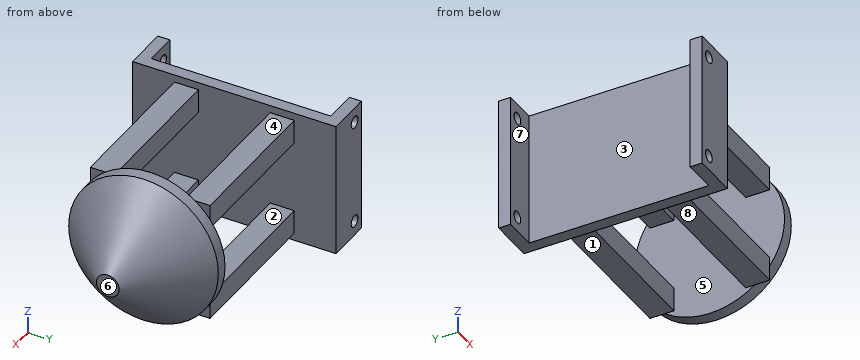
Autodesk Fusion 360 part; units mm, degrees
sketch "Sketch1" plane through (0, 0, 0) normal (0, 1, 0) x (1, 0, 0)
  line L0 (7.5, -22.5) -> (-7.5, -22.5)
  line L1 (-7.5, -22.5) -> (-7.5, 22.5)
  line L2 (-7.5, 22.5) -> (7.5, 22.5)
  line L3 (7.5, 22.5) -> (7.5, -22.5)
  line L4 (7.5, -22.5) -> (-7.5, 22.5) construction
  line L5 (-7.5, -22.5) -> (7.5, 22.5) construction
  dimension "d1" = 45
  dimension "d2" = 15
extrude "Extrude1" add sketch "Sketch1" along normal blind 4
sketch "Sketch2" plane through (0, 4, 0) normal (0, 1, 0) x (-1, 0, 0)
  line L0 (-7.5, -22.5) -> (7.5, -22.5)
  line L1 (7.5, -22.5) -> (7.5, 22.5)
  line L2 (7.5, 22.5) -> (-7.5, 22.5)
  line L3 (-7.5, 22.5) -> (-7.5, -22.5)
  line L4 (-7.5, 22.5) -> (-3.5, 22.5)
  line L5 (-3.5, 22.5) -> (-3.5, -22.5)
  line L6 (-3.5, -22.5) -> (-7.5, -22.5)
  line L7 (-7.5, -22.5) -> (-7.5, 22.5)
  dimension "d9" = 4
extrude "Extrude2" add sketch "Sketch2" along normal blind 64 contours L0 L2 L3 L4 L5 L6 L7
sketch "Sketch3" plane through (3.5, 0, 0) normal (-1, 0, 0) x (0, -1, 0)
  line L0 (-4, -22.5) -> (-4, 22.5)
  line L1 (-4, 22.5) -> (-68, 22.5)
  line L2 (-68, 22.5) -> (-68, -22.5)
  line L3 (-68, -22.5) -> (-4, -22.5)
  line L4 (-68, 22.5) -> (-64, 22.5)
  line L5 (-64, 22.5) -> (-64, -22.5)
  line L6 (-64, -22.5) -> (-68, -22.5)
  line L7 (-68, -22.5) -> (-68, 22.5)
  dimension "d12" = 4
extrude "Extrude3" add sketch "Sketch3" along normal blind 11 contours L1 L2 L3 L4 L5 L6 L7
sketch "Sketch4" plane through (3.5, 0, 0) normal (-1, 0, 0) x (0, -1, 0)
  line L0 (-64, 22.5) -> (-64, -22.5)
  line L1 (-64, -22.5) -> (-4, -22.5)
  line L2 (-4, -22.5) -> (-4, 22.5)
  line L3 (-4, 22.5) -> (-64, 22.5)
  line L4 (-60, 22.5) -> (-56, 22.5)
  line L5 (-56, 22.5) -> (-56, -22.5)
  line L6 (-56, -22.5) -> (-60, -22.5)
  line L7 (-60, -22.5) -> (-60, 22.5)
  line L8 (-34, -22.5) -> (-34, 22.5) construction
  line L9 (-8, 22.5) -> (-12, 22.5)
  line L10 (-8, -22.5) -> (-8, 22.5)
  line L11 (-12, 22.5) -> (-12, -22.5)
  line L12 (-12, -22.5) -> (-8, -22.5)
  dimension "d15" = 4
  dimension "d16" = 4
sketch "Sketch5" plane through (0, 68, 0) normal (0, 1, 0) x (-1, 0, 0)
  line L0 (-7.5, -22.5) -> (7.5, -22.5)
  line L1 (7.5, -22.5) -> (7.5, 22.5)
  line L2 (7.5, 22.5) -> (-7.5, 22.5)
  line L3 (-7.5, 22.5) -> (-7.5, -22.5)
  circle A0 centre (3.5, 17.4201) radius 2
  circle A1 centre (3.5, -17.5799) radius 2
  line L4 (3.5, -17.5799) -> (3.5, 17.4201) construction
  point P0 (3.5, -0.0799)
  dimension "d19" = 4
  dimension "d20" = 4
  dimension "d21" = 35
  dimension "d22" = 4
extrude "Extrude5" cut sketch "Sketch5" against normal through all contours A0 | A1
ref_plane "WorkPlane1" through (0, 34, 0) normal (0, 1, 0) x (0, 0, 1)
sketch "Sketch7" plane through (7.5, 0, 0) normal (1, 0, 0) x (0, 1, 0)
  line L0 (0, 22.5) -> (0, -22.5)
  line L1 (0, -22.5) -> (68, -22.5)
  line L2 (68, -22.5) -> (68, 22.5)
  line L3 (68, 22.5) -> (0, 22.5)
  line L4 (54, 20) -> (14, 20) construction
  line L5 (14, 20) -> (14, -20) construction
  line L6 (14, -20) -> (54, -20) construction
  line L7 (54, -20) -> (54, 20) construction
  line L8 (54, 20) -> (14, -20) construction
  line L9 (14, 20) -> (54, -20) construction
  line L10 (34, 22.5) -> (34, -22.5) construction
  line L11 (0, 0) -> (68, 0) construction
  line L12 (14, 20) -> (22, 20)
  line L13 (22, 20) -> (22, 12)
  line L14 (22, 12) -> (14, 12)
  line L15 (14, 12) -> (14, 20)
  line L16 (46, 12) -> (54, 12)
  line L17 (54, 12) -> (54, 20)
  line L18 (54, 20) -> (46, 20)
  line L19 (46, 20) -> (46, 12)
  line L20 (22, -12) -> (14, -12)
  line L21 (22, -20) -> (22, -12)
  line L22 (14, -20) -> (22, -20)
  line L23 (14, -12) -> (14, -20)
  line L24 (46, -20) -> (46, -12)
  line L25 (54, -20) -> (46, -20)
  line L26 (54, -12) -> (54, -20)
  line L27 (46, -12) -> (54, -12)
  point P0 (34, 0)
  dimension "d32" = 40
  dimension "d33" = 40
  dimension "d34" = 8
extrude "Extrude6" add sketch "Sketch7" along normal blind 50 contours L12 L13 L14 L15 | L16 L17 L18 L19 | L20 L21 L22 L23 | L24 L25 L26 L27
sketch "Sketch8" plane through (0, 34, 0) normal (0, 1, 0) x (1, 0, 0)
  line L0 (57.5, -20) -> (57.5, -12)
  line L1 (0, 0) -> (67.5, 0) construction
  line L2 (57.5, -25) -> (61.5, -25)
  line L3 (61.5, -25) -> (82.7132, -3.7868)
  line L4 (57.5, -25) -> (57.5, 0)
  line L5 (82.7132, -3.7868) -> (82.7132, 0)
  line L6 (82.7132, 0) -> (57.5, 0)
  point P0 (57.5, 0)
  dimension "d39" = 4
  dimension "d40" = 135
  dimension "d41" = 30
revolve "Revolve2" add sketch "Sketch8" angle 360 about axis through (0, 34, 0) along (1, 0, 0)
equation "d10 = 56 mm + 8 mm"
equation "d24 = -( 68 / 2 ) * 1 mm"
Here's how the part is built. I have some questions about the finished solid (model axes, mm). Face numbers are marked on the shaded views. A direction names the side the tool comes from. Round coordinates to 2 decimals unless told otherwise and drop trailing zeros. Loops run counter-clockwise (first coordinate to the right, second up) from the corner with the lowest first, then second, coordinate; pieces in that order, holes last. Notation, with made-up numbers: (25, 20) -> (63, 20) arc R11 cw to (63, 28) -> close; hole circle Ø3 at (74.25, -13.75). An arc over 180 degrees is marked (long way). Answer as CSV lines item,"result". Start each with the question number.
1. Imagine slicing it at D-D on x = -3.5. Write out the boundary of the cut face in (y, z), plus the area to 3 significant figures.
2. Imagine slicing it at A-A on x = 40. Write out the boundary of the cut face in (y, z), plus the area to 3 significant figures.
3. I'm going to push flat-ended pins straight in: P1, Ø12, axis at x = 19, z = -15, coming from the -Y side; P2, Ø4, axis at x = 32, y = 17.5, coming from the -Z side; P3, Ø2.5, axis at x = 30, y = 18.5, coming from the +Z side. Where does each tip first touch, or does it pass through?
4. I need wall thicknesses on probe 1 along Z at (x, y) = (-3.5, 1.75); probe 2 along Z at (x, y) = (12.5, 20.5); probe 3 along Y at (x, z) = (20, 14.5). Which ranges of each line are inside material? Lowest first, please. Write a range as from..to.
5. If we mould it in two halves opening along X, with no side actions, what happens to the marked faces 6, 7 and 8? For each: pulls with the +X half, pulls with the -X half, needs draft (parallel to the pull), parting line crosses it, or undercut.
6. Imagine slicing it at B-B on y = 34. Write out the boundary of the cut face in (x, z).
7. For the marked faces 1, 2, 3, 4 and 5, which set-ups out of +Z, -Z, +X, -X, +Y, -Y let a thin tool reach every point of the face, with its end or its side?
8. Imagine slicing it at C-C on z = 0. Write out the boundary of the cut face in (x, y).
Solution:
1,outline,"(0, -22.5) -> (4, -22.5) -> (4, -19.58) -> (0, -19.58) -> close; (0, -15.58) -> (4, -15.58) -> (4, 15.42) -> (0, 15.42) -> close; (0, 19.42) -> (4, 19.42) -> (4, 22.5) -> (0, 22.5) -> close; (64, -22.5) -> (68, -22.5) -> (68, -19.58) -> (64, -19.58) -> close; (64, -15.58) -> (68, -15.58) -> (68, 15.42) -> (64, 15.42) -> close; (64, 19.42) -> (68, 19.42) -> (68, 22.5) -> (64, 22.5) -> close"
1,area,"296 mm²"
2,outline,"(14, -20) -> (22, -20) -> (22, -12) -> (14, -12) -> close; (14, 12) -> (22, 12) -> (22, 20) -> (14, 20) -> close; (46, -20) -> (54, -20) -> (54, -12) -> (46, -12) -> close; (46, 12) -> (54, 12) -> (54, 20) -> (46, 20) -> close"
2,area,"256 mm²"
3,P1,"y = 14"
3,P2,"z = -20"
3,P3,"z = 20"
4,probe 1,"-22.5..-19.58, -15.58..15.42, 19.42..22.5"
4,probe 2,"-20..-12, 12..20"
4,probe 3,"14..22, 46..54"
5,face 6,"pulls with the +X half"
5,face 7,"needs draft"
5,face 8,"undercut"
6,outline,"(3.5, -22.5) -> (7.5, -22.5) -> (7.5, 22.5) -> (3.5, 22.5) -> close; (57.5, -25) -> (61.5, -25) -> (82.71, -3.79) -> (82.71, 3.79) -> (61.5, 25) -> (57.5, 25) -> close"
7,face 1,"-Z, +Y, -Y"
7,face 2,"+Y, -Y"
7,face 3,"+Z, -Z, -X"
7,face 4,"+Z, +Y, -Y"
7,face 5,"none"
8,outline,"(-7.5, 0) -> (7.5, 0) -> (7.5, 68) -> (-7.5, 68) -> (-7.5, 64) -> (3.5, 64) -> (3.5, 4) -> (-7.5, 4) -> close; (57.5, 9) -> (61.5, 9) -> (82.71, 30.21) -> (82.71, 37.79) -> (61.5, 59) -> (57.5, 59) -> close"
